The listing builds one solid part. Answer for the finished solid, in the listing's coordinates (mm). Coordinates: 2 decimals unless noted, no trailing zeros. Order: outer loops, then holes, each group sorted by start corner. A loop starts at its lowest first (then second) coordinate and runs counter-clockwise, first axis right, second up. Notation, with made-up numbers: (48.5, -32) -> (75.5, -32) arc R30 cw to (75.5, 6) -> close; hole circle Ø7 at (-12, -28.75). An arc over 180 degrees is marked (long way). Answer in a Markdown table with one row per item.
Autodesk Inventor part; units mm, degrees
ref_plane "YZ Plane" through (0, 0, 0) normal (1, 0, 0) x (0, 1, 0)
ref_plane "XZ Plane" through (0, 0, 0) normal (0, 1, 0) x (-1, 0, 0)
ref_plane "XY Plane" through (0, 0, 0) normal (0, 0, 1) x (1, 0, 0)
sketch "Sketch1" plane through (0, 0, 0) normal (0, 0, 1) x (1, 0, 0)
  line L0 (0, 0) -> (444.5, 0)
  line L1 (444.5, 0) -> (444.5, 127)
  line L2 (444.5, 127) -> (0, 127)
  line L3 (0, 127) -> (0, 0)
  dimension "d0" = 444.5
  dimension "d1" = 127
extrude "Extrusion1" add sketch "Sketch1" along normal blind 6.35
sketch "Sketch2" plane through (0, 0, 6.35) normal (0, 0, 1) x (1, 0, 0)
  line L0 (0, 0) -> (444.5, 0)
  line L1 (38.0923, 0) -> (0, 38.0919)
  line L2 (0, 127) -> (0, 0)
  line L3 (0, 0) -> (444.5, 0)
  line L4 (444.5, 0) -> (444.5, 127)
  line L5 (444.5, 0) -> (406.4, 0)
  line L6 (444.5, 0) -> (482.6, 0) construction
  line L7 (444.5, 0) -> (444.5, 38.0919)
  line L8 (444.5, 38.0919) -> (406.4086, 0)
  point P0 (419.1126, 0)
  dimension "d19" = 38.1
  dimension "d20" = 180
extrude "Extrusion2" cut sketch "Sketch2" against normal blind 50.8
sketch "Sketch3" plane through (0, 0, 6.35) normal (0, 0, 1) x (1, 0, 0)
  line L0 (0, 77.664) -> (80.645, 77.664) construction
  line L1 (444.5, 127) -> (0, 127)
  line L2 (80.645, 127) -> (161.29, 127) construction
  circle A0 centre (80.645, 46.355) radius 14.2748
  line L3 (444.5, 38.0919) -> (444.5, 127)
  line L4 (444.5, 77.664) -> (525.145, 77.664) construction
  line L5 (444.5, 38.0919) -> (444.5, 127)
  line L6 (444.5, 46.355) -> (525.145, 46.355) construction
  circle A1 centre (363.855, 46.355) radius 14.2748
  line L7 (444.5, 127) -> (0, 127)
  line L8 (0, 127) -> (0, 38.0919)
  circle A2 centre (182.245, 46.355) radius 21.59
  circle A3 centre (262.255, 46.355) radius 21.59
  point P0 (0, 0)
  dimension "d10" = 28.5496
  dimension "d18" = 28.5496
  dimension "d31" = 43.18
  dimension "d32" = 43.18
extrude "Extrusion3" cut sketch "Sketch3" against normal blind 50.8 contours A0 | A1
properties part number "MecanumDriveTrainPlate17-18"
(1) A cutting plane is placed at B-B, the plane y = 16. Determine the outline of the cut face in (x, z), then the cut area to 3 significant figures.
Check values:
| item | result |
|---|---|
| outline | (22.09, 0) -> (422.41, 0) -> (422.41, 6.35) -> (22.09, 6.35) -> close |
| area | 2,540 mm² |
(2) A cutting plane is placed at C-C, the plane x = 33.5. Determine the outline of the cut face in (y, z), then the cut area to 3 significant figures.
Check values:
| item | result |
|---|---|
| outline | (4.59, 0) -> (127, 0) -> (127, 6.35) -> (4.59, 6.35) -> close |
| area | 777 mm² |
(3) Find the intervals of material crossed by line 1 along X through (y, z) = (46, 1.75); line 2 along Y through (x, z) = (82.5, 3.5); line 3 along X through (y, z) = (56, 3), in increasing order. Write a range as from..to.
Check values:
| item | result |
|---|---|
| line 1 | 0..66.37, 94.92..349.58, 378.13..444.5 |
| line 2 | 0..32.2, 60.51..127 |
| line 3 | 0..70.12, 91.17..353.33, 374.38..444.5 |
(4) For a pull along X with two mould halves and no side action, classify faces 1 (the cylindrical face through (349.594, 46.983, 3.219)), 2 (the cylindrical face through (69.317, 37.669, 3.219)), 3 (the flat face through (425.72, 19.31, 3.22)), 4 (the flat face through (219, 64, 0)) as released by +X, released by -X, zero draft, split by the parting line, or undercut.
Check values:
| item | result |
|---|---|
| face 1 | undercut |
| face 2 | undercut |
| face 3 | released by +X |
| face 4 | zero draft |
(5) A cutting plane is placed at A-A, the plane z = 2.75. Determine the outline of the cut face in (x, y) (3 decimals), then the cut area to 3 significant figures.
Check values:
| item | result |
|---|---|
| outline | (0, 38.092) -> (38.092, 0) -> (406.409, 0) -> (444.5, 38.092) -> (444.5, 127) -> (0, 127) -> close; hole circle Ø28.55 at (80.645, 46.355); hole circle Ø28.55 at (363.855, 46.355) |
| area | 53,700 mm² |
